from build123d import *

# Parameters (mm, degrees)
BOSS_EXTRUDE1_START        = 8
SKETCH2_W                  = 381
SKETCH2_H                  = 2.032
BOSS_EXTRUDE1_DEPTH        = 37
SKETCH3_W                  = 345
SKETCH3_H                  = 2.032
BOSS_EXTRUDE2_DEPTH        = 10.668
SKETCH4_W                  = 40.623
SKETCH4_H                  = 17.5
CUT_EXTRUDE1_DEPTH         = 3
F_6_CLEARANCE_HOLE1_D      = 3.6576
FILLET2_R                  = 5
FILLET3_R                  = 3
SKETCH8_W                  = 2
SKETCH8_H                  = 4
CUT_EXTRUDE2_DEPTH         = 197.033303864
FLATTEN_BENDS1_START       = -11.684
FLATTEN_BENDS1_OUTLINE_W   = 345
FLATTEN_BENDS1_OUTLINE_H   = 2.032
FLATTEN_BENDS1_DEPTH       = 10.668
FLATTEN_BENDS1_START_2     = -1.016
FLATTEN_BENDS1_2_OUTLINE_W = 345
FLATTEN_BENDS1_2_OUTLINE_H = 9.367654589
FLATTEN_BENDS1_2_DEPTH     = 2.032
PROCESS_BENDS1_START       = -172.5
PROCESS_BENDS1_DEPTH       = 345
PROCESS_BENDS1_2_DEPTH     = 345


# Read off the part's stored shape, not the designer's step: Flatten-Bends1, Process-Bends1
with BuildPart() as part:
    # Sketch2 → Boss-Extrude1 (new body)
    with BuildSketch(Plane(origin=(0, 0, 0), x_dir=(1, 0, 0), z_dir=(0, 1, 0)).offset(BOSS_EXTRUDE1_START)):
        Rectangle(SKETCH2_W, SKETCH2_H)
    extrude(amount=BOSS_EXTRUDE1_DEPTH)

    # Sketch3 → Boss-Extrude2 (add)
    with BuildSketch(Plane(origin=(0, 0, -1.016), x_dir=(-1, 0, 0), z_dir=(0, 0, -1))):
        with Locations((0, 9.016)):
            Rectangle(SKETCH3_W, SKETCH3_H)
    extrude(amount=BOSS_EXTRUDE2_DEPTH)

    # Sketch4 → Cut-Extrude1 (cut)
    with BuildSketch(Plane.XY.offset(1.016)):
        with Locations((170.1885, 36.25)):
            Rectangle(SKETCH4_W, SKETCH4_H)
        with Locations((-170.1885, 36.25)):
            Rectangle(SKETCH4_W, SKETCH4_H)
    extrude(amount=-CUT_EXTRUDE1_DEPTH, mode=Mode.SUBTRACT)

    # #6 Clearance Hole1 (through all)
    with Locations(Plane.XY.offset(1.016)):
        with Locations((-121.9, 35), (-121.9, 19), (-85.5, 35), (-85.5, 19), (99.5, 19), (99.5, 35), (135.9, 35), (135.9, 19)):
            Hole(F_6_CLEARANCE_HOLE1_D / 2)

    # Fillet2
    fillet2_edges = [part.edges().sort_by_distance(p)[0] for p in [
        (-190.5, 27.5, 0),
        (-149.877, 45, 0),
        (190.5, 27.5, 0),
        (149.877, 45, 0),
        (-190.5, 8, 0),
        (190.5, 8, 0),
    ]]
    fillet(fillet2_edges, radius=FILLET2_R)

    # Fillet3
    fillet3_edges = [part.edges().sort_by_distance(p)[0] for p in [
        (-149.877, 27.5, 0),
        (149.877, 27.5, 0),
    ]]
    fillet(fillet3_edges, radius=FILLET3_R)

    # Sketch8 → Cut-Extrude2 (cut, through all)
    with BuildSketch(Plane(origin=(0, 0, -1.016), x_dir=(-1, 0, 0), z_dir=(0, 0, -1))):
        with Locations((173.5, 10)):
            Rectangle(SKETCH8_W, SKETCH8_H)
        with Locations((-173.5, 10)):
            Rectangle(SKETCH8_W, SKETCH8_H)
    extrude(amount=-CUT_EXTRUDE2_DEPTH, mode=Mode.SUBTRACT)

    # Flatten-Bends1 outline → Flatten-Bends1 (cut)
    with BuildSketch(Plane.XY.offset(FLATTEN_BENDS1_START)):
        with Locations((0, 9.016)):
            Rectangle(FLATTEN_BENDS1_OUTLINE_W, FLATTEN_BENDS1_OUTLINE_H)
    extrude(amount=FLATTEN_BENDS1_DEPTH, mode=Mode.SUBTRACT)

    # Flatten-Bends1 2 outline → Flatten-Bends1 2 (add)
    with BuildSketch(Plane.XY.offset(FLATTEN_BENDS1_START_2)):
        with Locations((0, 3.316172706)):
            Rectangle(FLATTEN_BENDS1_2_OUTLINE_W, FLATTEN_BENDS1_2_OUTLINE_H)
    extrude(amount=FLATTEN_BENDS1_2_DEPTH)

    # Process-Bends1 outline → Process-Bends1 (cut)
    with BuildSketch(Plane.YZ.offset(PROCESS_BENDS1_START)):
        with BuildLine():
            Line((-1.367654589, -1.016), (8.254000001, -1.016))
            ThreePointArc((8.254000001, -1.016), (9.470379953, 0.461430071), (11.302, 1.016))
            Line((11.302, 1.016), (-1.367654589, 1.016))
            Line((-1.367654589, 1.016), (-1.367654589, -1.016))
        make_face()
    extrude(amount=PROCESS_BENDS1_DEPTH, mode=Mode.SUBTRACT)

    # Process-Bends1 2 outline → Process-Bends1 2 (add)
    with BuildSketch(Plane.YZ.offset(PROCESS_BENDS1_START)):
        with BuildLine():
            Line((8, -2.286), (8, -11.684))
            Line((8, -11.684), (10.032, -11.684))
            Line((10.032, -11.684), (10.032, -2.286))
            ThreePointArc((10.032, -2.286), (10.403974388, -1.387974388), (11.302, -1.016))
            Line((11.302, -1.016), (8.254000001, -1.016))
            ThreePointArc((8.254000001, -1.016), (8.064122609, -1.638424522), (8, -2.286))
        make_face()
    extrude(amount=PROCESS_BENDS1_2_DEPTH)


solid = part.part
Verification items for the finished model (mm, model axes). A direction names the side the tool comes from. Give positions to 0.01 mm unless a question says otherwise; leave off trailing zeros. Loops run counter-clockwise (first coordinate to the right, second up) from the corner with the lowest first, then second, coordinate; pieces in that order, holes last.
1) Set-up check for faces 1 (the flat face through (-2, 10.032, -7)), 2 (the flat face through (-2, 8, -7)): record each of +Z, -Z, +X, -X, +Y, -Y from which the full face is reachable in a straight line by a thin tool's end or side.
2) Thickness scan on line 1 along Y through (x, z) = (-121.9, 0.55); line 2 along X through (y, z) = (34, -0.25); line 3 along Y through (x, z) = (-121.9, -0.3). Record the ranges inside material, lowest first.
3) Sectioned sample at A-A, the plane x = 4.5. Enter the section's corners in (y, z), then the cut area to 3 significant figures.
4) Depth check by flat-ended pin: pin 1 Ø2 at (x, z) = (-169, -0.5) entering from +Y; pin 2 Ø1.6 at (y, z) = (37.5, 0) entering from -X; pin 3 Ø4 at (x, z) = (97.5, -9.5) entering from +Y. Enter the tip coordinate at first touch or a pass-through.
5) Sectioned sample at B-B, the plane z = -4.25. Enter the section's corners in (x, y).
Answers:
1. face 1: -Z, +X, -X, +Y
1. face 2: +Z, -Z, +X, -X, -Y
2. line 1: y = 9.61 to 17.17, 20.83 to 33.17, 36.83 to 45
2. line 2: x = -149.88 to -123.43, -120.37 to -87.03, -83.97 to 97.97, 101.03 to 134.37, 137.43 to 149.88
2. line 3: y = 8.66 to 17.17, 20.83 to 33.17, 36.83 to 45
3. outline: (8, -11.68) - (10.03, -11.68) - (10.03, -2.29) arc R1.27 cw to (11.3, -1.02) - (45, -1.02) - (45, 1.02) - (11.3, 1.02) arc R3.3 ccw to (8, -2.29) - close
3. area: 94.9 mm2
4. pin 1: stops at y = 27.5
4. pin 2: stops at x = -149.88
4. pin 3: stops at y = 10.03
5. outline: (-172.5, 8) - (172.5, 8) - (172.5, 10.03) - (-172.5, 10.03) - close
